Can you work these out from the drawing? Everything is in mm from the part's minimum corner. A direction names the side the tool comes from. Coordinates: 2 decimals unless noted, no trailing zeros. Write each loop counter-clockwise with the first axis right and the second up, starting at its lowest first coordinate (ties: lowest second). Pieces come first, ordered by that corner, then holes. Notation, with made-up numbers: M 8.25,38 L 19.25,38 A23 ccw 19.25,73 Z; hole C 69,-28.5 d5. An arc over 180 degrees is marked long. Write item = value, one per line.
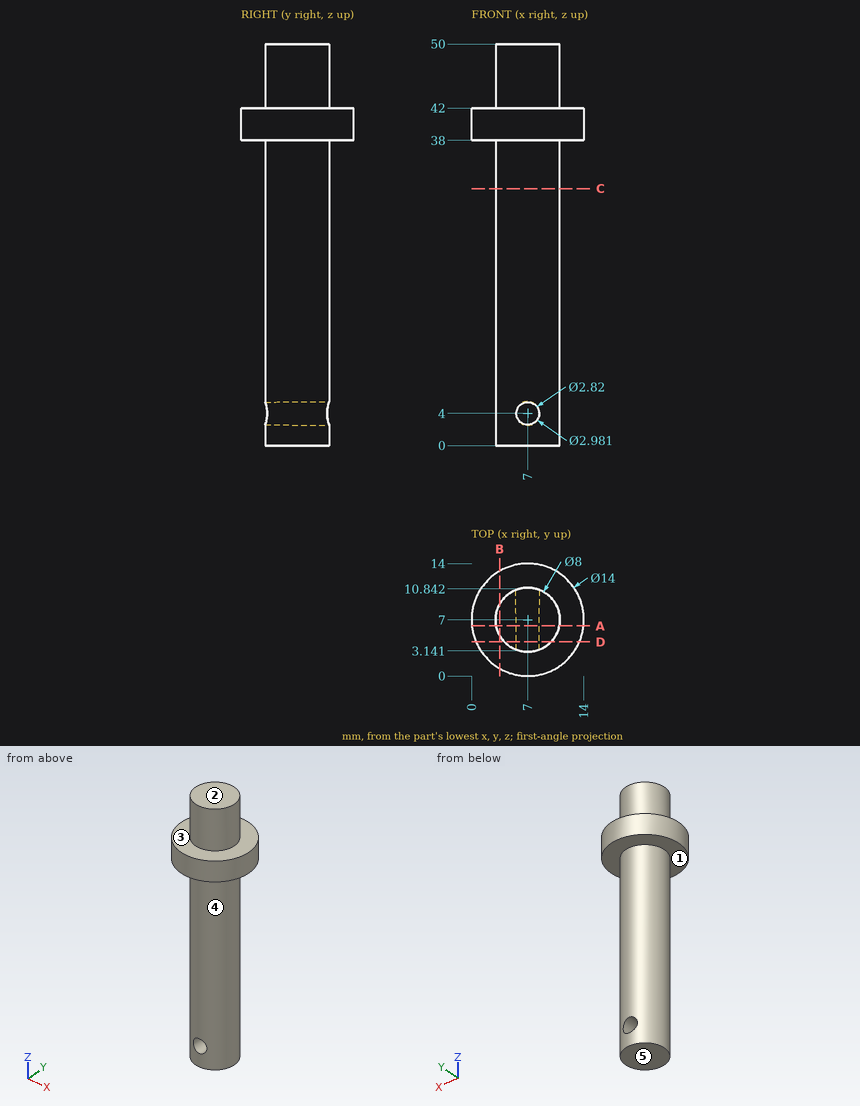
Item 1: Imagine slicing it at A-A (y = 6.25). Write out the boundary of the cut face in (x, z) (1 decimal).
Numbers:
outline = M 0,38 L 3.1,38 L 3.1,0 L 10.9,0 L 10.9,38 L 14,38 L 14,42 L 10.9,42 L 10.9,50 L 3.1,50 L 3.1,42 L 0,42 Z; hole C 7,4 d2.9
Item 2: If I drill on line 1 along Z through (x, y) = (7.25, 11.5); line 2 along X through (y, z) = (6.5, 43); line 3 along X through (y, z) = (8.75, 7) (1 decimal), over which ranges is the centre line in solid material (lowest first)?
Numbers:
line_1 = 38 to 42
line_2 = 3.03 to 10.97
line_3 = 3.4 to 10.6
Item 3: For the marked faces 1, 2 and 3, which set-ups out of +Z, -Z, +X, -X, +Y, -Y let a thin tool reach every point of the face, with its end or its side?
Numbers:
face_1 = -Z
face_2 = +Z, +X, -X, +Y, -Y
face_3 = +Z
Item 4: Imagine slicing it at B-B (x = 3.5). Write out the boundary of the cut face in (y, z), and give its area (3 significant figures).
Numbers:
outline = M 0.94,38 L 5.06,38 L 5.06,0 L 8.94,0 L 8.94,38 L 13.06,38 L 13.06,42 L 8.94,42 L 8.94,50 L 5.06,50 L 5.06,42 L 0.94,42 Z
area = 227 mm²
Item 5: Imagine slicing it at C-C (z = 32). Write out the boundary of the cut face in (x, y).
Numbers:
outline = C 7,7 d8
Item 6: I'm going to push flat-ended pins straight in: P1, Ø4, axis at y = 5.5, z = 9, coming from the +X side; P2, Ø1, axis at y = 5.5, z = 12, coming from the +X side; P3, Ø4, axis at x = 11.5, z = 28.5, coming from the +Y side. Where does each tip first touch, or does it pass through?
Numbers:
P1 = 11
P2 = 10.87
P3 = 10.12
Item 7: Imagine slicing it at D-D (y = 4.25). Write out the boundary of the cut face in (x, z) (1 decimal).
Numbers:
outline = M 0.6,38 L 4.1,38 L 4.1,0 L 9.9,0 L 9.9,38 L 13.4,38 L 13.4,42 L 9.9,42 L 9.9,50 L 4.1,50 L 4.1,42 L 0.6,42 Z; hole C 7,4 d2.8
Item 8: If we mould it in two halves opening along Y, with no side actions, what happens to the marked faces 4 and 5? For each: pulls with the +Y half, pulls with the -Y half, needs draft (parallel to the pull), parting line crosses it, or undercut.
Numbers:
face_4 = parting line crosses it
face_5 = needs draft
